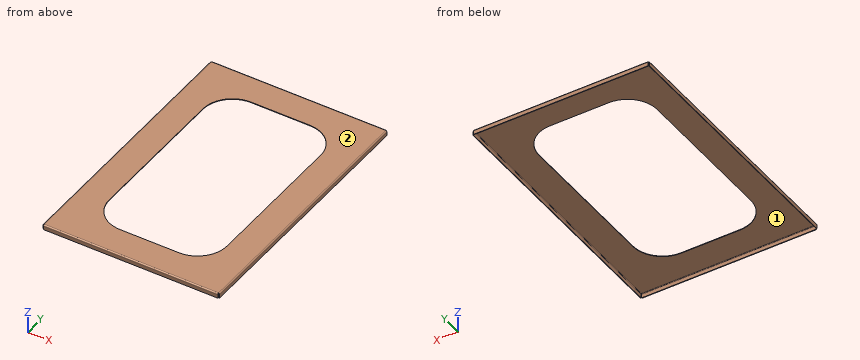
Autodesk Inventor part; units mm, degrees
ref_plane "YZ Plane" through (0, 0, 0) normal (1, 0, 0) x (0, 1, 0)
ref_plane "XZ Plane" through (0, 0, 0) normal (0, 1, 0) x (-1, 0, 0)
ref_plane "XY Plane" through (0, 0, 0) normal (0, 0, 1) x (1, 0, 0)
sketch "Sketch1" plane through (0, 0, 0) normal (0, 0, 1) x (1, 0, 0)
  line L0 (-450, -675) -> (450, -675)
  line L1 (450, -675) -> (450, 675)
  line L2 (450, 675) -> (-450, 675)
  line L3 (-450, 675) -> (-450, -675)
  line L4 (-450, -675) -> (450, 675) construction
  line L5 (450, -675) -> (-450, 675) construction
  line L6 (-150, 525) -> (150, 525)
  line L7 (300, 375) -> (300, -375)
  line L8 (150, -525) -> (-150, -525)
  line L9 (-300, -375) -> (-300, 375)
  arc A0 (300, 375) -> (150, 525) centre (150, 375) ccw
  arc A1 (-150, 525) -> (-300, 375) centre (-150, 375) ccw
  arc A2 (-300, -375) -> (-150, -525) centre (-150, -375) ccw
  arc A3 (150, -525) -> (300, -375) centre (150, -375) ccw
  point P0 (0, 0)
  dimension "d0" = 900
  dimension "d1" = 1350
  dimension "d13" = 150
  dimension "d14" = 150
  dimension "d15" = 150
  dimension "d16" = 150
  dimension "d17" = 150
extrude "Plate3" add sketch "Sketch1" along normal blind 3.048
sketch "Sketch3" plane through (450, 671.952, 3.048) normal (0, 1, 0) x (-1, 0, 0)
  line L0 (900, 0) -> (0, 0)
  line L1 (0, 0) -> (0, -25)
  line L2 (0, -25) -> (900, -25)
  line L3 (900, -25) -> (900, 0)
edge flange "Flange2" height 25 angle 90 thickness 3.048 bend radius 3.048 thickness toward (0, 1, 0) relief tear relief width 3.048 relief depth 1.524 corner gap 3.048 corner form 2 edges at (0, 675, 0) (-450, 0, 0) (450, 0, 0) (0, -675, 0) wall of the first edge with corners at (-450, 671.952, 3.048) (450, 671.952, 3.048) (450, 671.952, -21.952) (-450, 671.952, -21.952)
bend "Bend2"
corner "Corner2"
equation "\"d18\" = Thickness"
equation "\"d19\" = BendReliefWidth"
equation "\"d20\" = BendReliefDepth"
equation "\"d21\" = MinimumRemnant"
equation "\"d22\" = TransitionRadius"
equation "\"d25\" = BendRadius"
equation "\"d26\" = CornerReliefSize"
equation "\"d27\" = GapSize"
equation "\"d28\" = JacobiRadiusSize"
equation "\"BendRadius\" = Thickness"
equation "\"BendReliefWidth\" = Thickness"
equation "\"BendReliefDepth\" = 0.5 * Thickness"
equation "\"CornerReliefSize\" = 4 * Thickness"
equation "\"MinimumRemnant\" = 2 * Thickness"
equation "\"TransitionRadius\" = BendRadius"
equation "\"JacobiRadiusSize\" = BendRadius"
equation "\"GapSize\" = Thickness"
equation "\"Space5\" = 0"
equation "\"Space6\" = 0"
equation "\"Space7\" = 0"
properties part number "TapaCentral"
For this review, take the finished solid that the model builds, in its own axes (mm). Face numbers are marked on the shaded views. Round coordinates to 2 decimals unless told otherwise and drop trailing zeros. Write each loop counter-clockwise with the first axis right and the second up, starting at its lowest first coordinate (ties: lowest second). Pieces come first, ordered by that corner, then holes. Notation, with made-up numbers: (82.5, 79.25) - (133.5, 79.25) arc R12 cw to (133.5, 99.25) - close; hole circle Ø4 at (57, 26.5). An arc over 180 degrees is marked (long way). Use a Markdown table: item, result.
Q1. We need section A-A (x = -102). Give the boundary of the cut face in (y, z), plus the area to 3 significant figures.
Derived:
| item | result |
|---|---|
| outline | (-675, -21.95) - (-671.95, -21.95) - (-671.95, -3.05) arc R3.05 cw to (-668.9, 0) - (-525, 0) - (-525, 3.05) - (-668.9, 3.05) arc R6.1 ccw to (-675, -3.05) - close; (525, 0) - (668.9, 0) arc R3.05 cw to (671.95, -3.05) - (671.95, -21.95) - (675, -21.95) - (675, -3.05) arc R6.1 ccw to (668.9, 3.05) - (525, 3.05) - close |
| area | 1,040 mm2 |
Q2. We need section B-B (y = -234.5). Give the boundary of the cut face in (x, z).
Derived:
| item | result |
|---|---|
| outline | (-450, -21.95) - (-446.95, -21.95) - (-446.95, -3.05) arc R3.05 cw to (-443.9, 0) - (-300, 0) - (-300, 3.05) - (-443.9, 3.05) arc R6.1 ccw to (-450, -3.05) - close; (300, 0) - (443.9, 0) arc R3.05 cw to (446.95, -3.05) - (446.95, -21.95) - (450, -21.95) - (450, -3.05) arc R6.1 ccw to (443.9, 3.05) - (300, 3.05) - close |
Q3. Wall thickness on line 1 along X through (y, z) = (-229.5, -17.25); line 2 along Y through (x, z) = (-73.5, -1.75); line 3 along Y through (x, z) = (-398.5, -17.25): over which ranges is each line inside the solid? List them lowest first.
Derived:
| item | result |
|---|---|
| line 1 | x = -450 to -446.95, 446.95 to 450 |
| line 2 | y = -674.86 to -671.66, 671.66 to 674.86 |
| line 3 | y = -675 to -671.95, 671.95 to 675 |
Q4. We need section C-C (z = -15.75). Give the boundary of the cut face in (x, y), plus the area to 3 significant figures.
Derived:
| item | result |
|---|---|
| outline | (-450, -669.8) - (-446.95, -669.8) - (-446.95, 669.8) - (-450, 669.8) - close; (-444.8, -675) - (444.8, -675) - (444.8, -671.95) - (-444.8, -671.95) - close; (-444.8, 671.95) - (444.8, 671.95) - (444.8, 675) - (-444.8, 675) - close; (446.95, -669.8) - (450, -669.8) - (450, 669.8) - (446.95, 669.8) - close |
| area | 13,600 mm2 |
Q5. The part is to be moulded in two halves that separate along X. For the marked faces 1 and 2, say which applies: pulls with the +X half, pulls with the -X half, needs draft (parallel to the pull), parting line crosses it, or undercut.
Derived:
| item | result |
|---|---|
| face 1 | undercut |
| face 2 | needs draft |
Q6. We need section D-D (x = 330). Give the boundary of the cut face in (y, z), plus the area to 3 significant figures.
Derived:
| item | result |
|---|---|
| outline | (-675, -21.95) - (-671.95, -21.95) - (-671.95, -3.05) arc R3.05 cw to (-668.9, 0) - (668.9, 0) arc R3.05 cw to (671.95, -3.05) - (671.95, -21.95) - (675, -21.95) - (675, -3.05) arc R6.1 ccw to (668.9, 3.05) - (-668.9, 3.05) arc R6.1 ccw to (-675, -3.05) - close |
| area | 4,240 mm2 |
Q7. Clearance check with flat-ended pins moving along their axes: pin 1 (2.5 mm diameter, centred on y = 673.5, z = -17, fed in from +X); pin 2 (10 mm diameter, centred on x = -349.5, y = 117.5, fed in from -Z); pin 3 (1.8 mm diameter, centred on x = -448, z = -1.5, fed in from +Y). State where each tip first meets the part, or that it passes through.
Derived:
| item | result |
|---|---|
| pin 1 | stops at x = 444.8 |
| pin 2 | stops at z = 0 |
| pin 3 | stops at y = 668.9 |
